For this review, take the finished solid that the model builds, in its own axes (mm). A direction names the side the tool comes from. Give positions to 0.01 mm unless a question says otherwise; leave off trailing zeros. Order: outer loops, then holes, each group sorted by start corner. A loop starts at its lowest first (then second) coordinate and runs counter-clockwise, first axis right, second up.
from build123d import *


with BuildPart() as part:
    # Sketch6 → Revolve1 (revolve)
    with BuildSketch(Plane.XY, mode=Mode.PRIVATE) as revolve1_sk:
        with BuildLine():
            Line((337.5, 165), (337.5, 200))
            Line((337.5, 200), (352.5, 200))
            Line((352.5, 200), (352.5, 180))
            Line((352.5, 180), (490, 180))
            ThreePointArc((490, 180), (500.606601718, 175.606601718), (505, 165))
            Line((505, 165), (505, 0))
            Line((505, 0), (505, -70))
            Line((505, -70), (490, -70))
            Line((490, -70), (490, 0))
            Line((490, 0), (490, 165))
            Line((490, 165), (337.5, 165))
        make_face()
    revolve(revolve1_sk.sketch.rotate(Axis((0, 0, 0), (0, 1, 0)), 90), axis=Axis((0, 0, 0), (0, 1, 0)))


solid = part.part
1) Tool access review of faces 1 (the face through (434.71, 49.14, -226.11)), 2 (the face through (181, 200, 286)), 3 (the face through (-116, 180, -334)): name each direction out of +Z, -Z, +X, -X, +Y, -Y from which nothing blocks a thin tool from reaching the whole face with its end or side.
Answer sheet:
face 1: -Y
face 2: +Z, -Z, +X, -X, +Y
face 3: +Y
2) To check wall thickness, follow line 1 (X direction, y = -14.5, z = 0); line 2 (X direction, y = 185, z = 0); line 3 (Y direction, x = -318.5, z = -375). State the ranges of each line that lie inside material, in increasing order.
Answer sheet:
line 1: x = -505 to -490, 490 to 505
line 2: x = -352.5 to -337.5, 337.5 to 352.5
line 3: y = -70 to 179.87
3) We need section C-C on y = 62. Give the boundary of the cut face in (x, z).
Answer sheet:
outline: circle Ø1010 at (0, 0); hole circle Ø980 at (0, 0)
4) We need section B-B on z = 0. Give the boundary of the cut face in (x, y), then the cut area to 3 significant figures.
Answer sheet:
outline: (-505, -70) - (-490, -70) - (-490, 165) - (-337.5, 165) - (-337.5, 200) - (-352.5, 200) - (-352.5, 180) - (-490, 180) arc R15 ccw to (-505, 165) - close; (337.5, 165) - (490, 165) - (490, -70) - (505, -70) - (505, 165) arc R15 ccw to (490, 180) - (352.5, 180) - (352.5, 200) - (337.5, 200) - close
area: 12,600 mm2
5) We need section A-A on x = 0. Give the boundary of the cut face in (y, z).
Answer sheet:
outline: (-70, -505) - (165, -505) arc R15 ccw to (180, -490) - (180, -352.5) - (200, -352.5) - (200, -337.5) - (165, -337.5) - (165, -490) - (-70, -490) - close; (-70, 490) - (165, 490) - (165, 337.5) - (200, 337.5) - (200, 352.5) - (180, 352.5) - (180, 490) arc R15 ccw to (165, 505) - (-70, 505) - close
6) Clearance check with flat-ended pins moving along their axes: pin 1 (8 mm diameter, centred on x = 136.5, y = 13, fed in from +Z); pin 2 (1.5 mm diameter, centred on x = -147.5, y = 110.5, fed in from -Z); pin 3 (1.5 mm diameter, centred on y = 13.5, z = -87.5, fed in from +X). State where each tip first meets the part, or that it passes through.
Answer sheet:
pin 1: stops at z = 487.31
pin 2: stops at z = -483.21
pin 3: stops at x = 497.49
7) Draft analysis for pull direction Z (two halves, no side actions). For faces 4 (the face through (344.118, 189.86, 76.415)), 5 (the face through (-334.628, 182.745, 43.936)), 6 (the face through (-264, -70, 414)), 7 (the face through (320, 165, 116)), state which applies: +Z half, -Z half, draft (parallel to the pull), parting line (faces both ways), or undercut.
Answer sheet:
face 4: parting line
face 5: undercut
face 6: draft
face 7: undercut
